Can you work these out from the model? Positions are in its coordinate system, mm. A direction names the side the tool comes from. Round coordinates to 2 decimals unless told otherwise and drop trailing zeros. Loops run counter-clockwise (first coordinate to the right, second up) from the corner with the lowest first, then second, coordinate; pieces in that order, holes last. Notation, with made-up numbers: (-5, 65.5) -> (0, 65.5) arc R21 ccw to (0, 82.5) -> close; hole circle Ø4 at (66.5, 46.5). An arc over 180 degrees is marked (long way). Answer as a JSON object with one key per item and string values.
```python
from build123d import *

# Parameters (mm, degrees)
SKETCH2_R           = 0.75
BOSS_EXTRUDE1_DEPTH = 2


with BuildPart() as part:
    # Sketch2 → Boss-Extrude1 (new body)
    with BuildSketch(Plane.XY):
        with BuildLine():
            Line((0, 7), (0, 12.455))
            Line((0, 12.455), (4, 12.455))
            Line((4, 12.455), (4, 14.455))
            Line((4, 14.455), (0, 14.455))
            Line((0, 14.455), (0, 17.455))
            ThreePointArc((0, 17.455), (0.585786438, 18.869213562), (2, 19.455))
            Line((2, 19.455), (14.2, 19.455))
            ThreePointArc((14.2, 19.455), (15.614213562, 18.869213562), (16.2, 17.455))
            Line((16.2, 17.455), (16.2, 14.455))
            Line((16.2, 14.455), (12.2, 14.455))
            Line((12.2, 14.455), (12.2, 12.455))
            Line((12.2, 12.455), (16.2, 12.455))
            Line((16.2, 12.455), (16.2, 7))
            Line((16.2, 7), (12.2, 7))
            Line((12.2, 7), (12.2, 5))
            Line((12.2, 5), (16.2, 5))
            Line((16.2, 5), (16.2, 2))
            ThreePointArc((16.2, 2), (15.614213562, 0.585786438), (14.2, 0))
            Line((14.2, 0), (2, 0))
            ThreePointArc((2, 0), (0.585786438, 0.585786438), (0, 2))
            Line((0, 2), (0, 5))
            Line((0, 5), (4, 5))
            Line((4, 5), (4, 7))
            Line((4, 7), (0, 7))
        make_face()
        with Locations((13.45, 2.5)):
            Circle(SKETCH2_R, mode=Mode.SUBTRACT)
        with Locations((2.75, 16.955)):
            Circle(SKETCH2_R, mode=Mode.SUBTRACT)
        with Locations((2.75, 2.5)):
            Circle(SKETCH2_R, mode=Mode.SUBTRACT)
        with Locations((13.45, 16.955)):
            Circle(SKETCH2_R, mode=Mode.SUBTRACT)
    extrude(amount=BOSS_EXTRUDE1_DEPTH)


solid = part.part
```
Q1. I want a section at D-D, the plane z = 1.4. Write out the boundary of the cut face in (x, y) (3 decimals).
Determined:
{"outline": "(0, 2) arc R2 ccw to (2, 0) -> (14.2, 0) arc R2 ccw to (16.2, 2) -> (16.2, 5) -> (12.2, 5) -> (12.2, 7) -> (16.2, 7) -> (16.2, 12.455) -> (12.2, 12.455) -> (12.2, 14.455) -> (16.2, 14.455) -> (16.2, 17.455) arc R2 ccw to (14.2, 19.455) -> (2, 19.455) arc R2 ccw to (0, 17.455) -> (0, 14.455) -> (4, 14.455) -> (4, 12.455) -> (0, 12.455) -> (0, 7) -> (4, 7) -> (4, 5) -> (0, 5) -> close; hole circle Ø1.5 at (2.75, 2.5); hole circle Ø1.5 at (2.75, 16.955); hole circle Ø1.5 at (13.45, 2.5); hole circle Ø1.5 at (13.45, 16.955)"}
Q2. I'm going to push a flat-ended pin straight in: pin 1 (0.6 mm diameter, centred on x = 15, z = 0.5, fed in from +Y). Where does the tip first touch, or does it pass through?
Determined:
{"pin 1": "y = 19.39"}
Q3. I want a section at B-B, the plane x = 3.75. Write out the boundary of the cut face in (y, z) (3 decimals), then the cut area to 3 significant figures.
Determined:
{"outline": "(0, 0) -> (5, 0) -> (5, 2) -> (0, 2) -> close; (7, 0) -> (12.455, 0) -> (12.455, 2) -> (7, 2) -> close; (14.455, 0) -> (19.455, 0) -> (19.455, 2) -> (14.455, 2) -> close", "area": "30.9 mm²"}
Q4. We'd pull the mould along X, two halves only. Please class faces 1 (the cylindrical face through (0.6, 0.57, 0.99)), 2 (the cylindrical face through (14.165, 2.725, 0.986)), 3 (the cylindrical face through (15.63, 0.6, 0.99)): pulls with the +X half, pulls with the -X half, needs draft (parallel to the pull), parting line crosses it, or undercut.
Determined:
{"face 1": "pulls with the -X half", "face 2": "undercut", "face 3": "pulls with the +X half"}
Q5. I want a section at C-C, the plane x = 13.45. Write out the boundary of the cut face in (y, z) (3 decimals).
Determined:
{"outline": "(0, 0) -> (1.75, 0) -> (1.75, 2) -> (0, 2) -> close; (3.25, 0) -> (5, 0) -> (5, 2) -> (3.25, 2) -> close; (7, 0) -> (12.455, 0) -> (12.455, 2) -> (7, 2) -> close; (14.455, 0) -> (16.205, 0) -> (16.205, 2) -> (14.455, 2) -> close; (17.705, 0) -> (19.455, 0) -> (19.455, 2) -> (17.705, 2) -> close"}
Q6. On a 3-axis mill with a long thin cutter (end or side, diameter ignored), from which of +Z, -Z, +X, -X, +Y, -Y can I reach the whole of each face in a straight line? I mean faces 4 (the flat face through (2, 7, 1)), 5 (the cylindrical face through (0.57, 18.854, 0.986)), 6 (the flat face through (14, 12.455, 1)). Say none if no direction works.
Determined:
{"face 4": "+Z, -Z, -X", "face 5": "+Z, -Z, -X, +Y", "face 6": "+Z, -Z, +X"}
Q7. I want a section at A-A, the plane y = 2.5. Write out the boundary of the cut face in (x, z), then the cut area to 3 significant figures.
Determined:
{"outline": "(0, 0) -> (2, 0) -> (2, 2) -> (0, 2) -> close; (3.5, 0) -> (12.7, 0) -> (12.7, 2) -> (3.5, 2) -> close; (14.2, 0) -> (16.2, 0) -> (16.2, 2) -> (14.2, 2) -> close", "area": "26.4 mm²"}
Q8. If I drill on L1, parallel to Y at x = 2.75, z = 0.65 (3 decimals); L2, parallel to X at y = 17.25, z = 0.5; L3, parallel to Y at x = 3.25, z = 1.4 (3 decimals), over which ranges is the centre line in solid material (lowest first)? Write a range as [from, to].
Determined:
{"L1": "[0, 1.75], [3.25, 5], [7, 12.455], [14.455, 16.205], [17.705, 19.455]", "L2": "[0, 2.06], [3.44, 12.76], [14.14, 16.2]", "L3": "[0, 1.941], [3.059, 5], [7, 12.455], [14.455, 16.396], [17.514, 19.455]"}
